from build123d import *

# Parameters (mm, degrees)
F0_W     = 10
F0_H     = 10
F0_W_2   = 8
F0_H_2   = 8
F1_DEPTH = 55
F2_R     = 1.5
F3_DEPTH = 25
F4_R     = 1.5
F5_DEPTH = 25


with BuildPart() as f1:
    # F0 (on Right) → F1 (new body)
    with BuildSketch(Plane.YZ):
        Rectangle(F0_W, F0_H)
        Rectangle(F0_W_2, F0_H_2, mode=Mode.SUBTRACT)
    extrude(amount=F1_DEPTH)

    # F2 (on face) → F3 (cut)
    with BuildSketch(Plane.XY.offset(5)):
        with Locations((5, 0)):
            Circle(F2_R)
        with Locations((50, 0)):
            Circle(F2_R)
    extrude(amount=-F3_DEPTH, mode=Mode.SUBTRACT)

    # F4 (on face) → F5 (cut)
    with BuildSketch(Plane.XZ.offset(5)):
        with Locations((15, 0)):
            Circle(F4_R)
        with Locations((40, 0)):
            Circle(F4_R)
    extrude(amount=-F5_DEPTH, mode=Mode.SUBTRACT)


solid = f1.part
Read the model definition and answer for the solid it produces. Units are mm, in the model's axes. A direction names the side the tool comes from. Give positions to 0.01 mm unless a question says otherwise; leave off trailing zeros. Write each loop counter-clockwise with the first axis right and the second up, starting at its lowest first coordinate (ties: lowest second). Pieces come first, ordered by that corner, then holes. Notation, with made-up numbers: (50.5, 55) - (91.5, 55) arc R15 cw to (91.5, 79) - close; hole circle Ø7 at (58.25, 57). An arc over 180 degrees is marked (long way). Use CSV: the item, a comma, the result in double quotes. Start each with the question number.
(1) Determine the mould class of faces 1 (the flat face through (27, -5, 0)), 2 (the cylindrical face through (13.5, 4.49, 0.07)), 3 (the flat face through (27, 0, 5)) for opening direction Z: +Z half, -Z half, draft (parallel to the pull), parting line (faces both ways), or undercut.
(2) Find section A-A (z = 0). Give the vertices of the cut face in (x, y).
(3) For faces 4 (the flat face through (27, 4, 0)), 5 (the flat face through (27, 0, -5)), determine the directions among +Z, -Z, +X, -X, +Y, -Y from which every point of the face is accessible in a straight line to the end or side of a thin tool.
(4) Find section B-B (x = 50). Give the vertices of the cut face in (y, z), plus the area to 3 significant figures.
(5) Given P1, Ø1.8, axis at x = 40, z = 0, coming from the -Y side, flat-ended and moving along its own axis, determine where the tip first touches the part or whether it passes through.
(6) Find section C-C (y = 0). Give the vertices of the cut face in (x, z).
(7) Find section D-D (z = -3). Give the vertices of the cut face in (x, y).
(8) Consider line 1 along Z through (x, y) = (34, 0); line 2 along X through (y, z) = (0.5, -4.25); line 3 along Z through (x, y) = (15, -4.5). Determine where each line is inside the solid, lowest interval first.
Findings below:
1,face 1,"draft"
1,face 2,"undercut"
1,face 3,"+Z half"
2,outline,"(0, -5) - (13.5, -5) - (13.5, -4) - (0, -4) - close; (0, 4) - (13.5, 4) - (13.5, 5) - (0, 5) - close; (16.5, -5) - (38.5, -5) - (38.5, -4) - (16.5, -4) - close; (16.5, 4) - (38.5, 4) - (38.5, 5) - (16.5, 5) - close; (41.5, -5) - (55, -5) - (55, -4) - (41.5, -4) - close; (41.5, 4) - (55, 4) - (55, 5) - (41.5, 5) - close"
3,face 4,"+X, -X"
3,face 5,"-Z, +X, -X, +Y, -Y"
4,outline,"(-5, -5) - (-1.5, -5) - (-1.5, -4) - (-4, -4) - (-4, 4) - (-1.5, 4) - (-1.5, 5) - (-5, 5) - close; (1.5, -5) - (5, -5) - (5, 5) - (1.5, 5) - (1.5, 4) - (4, 4) - (4, -4) - (1.5, -4) - close"
4,area,"30.0 mm2"
5,P1,"through"
6,outline,"(0, -5) - (3.5, -5) - (3.5, -4) - (0, -4) - close; (0, 4) - (3.5, 4) - (3.5, 5) - (0, 5) - close; (6.5, -5) - (48.5, -5) - (48.5, -4) - (6.5, -4) - close; (6.5, 4) - (48.5, 4) - (48.5, 5) - (6.5, 5) - close; (51.5, -5) - (55, -5) - (55, -4) - (51.5, -4) - close; (51.5, 4) - (55, 4) - (55, 5) - (51.5, 5) - close"
7,outline,"(0, -5) - (55, -5) - (55, -4) - (0, -4) - close; (0, 4) - (55, 4) - (55, 5) - (0, 5) - close"
8,line 1,"-5 to -4, 4 to 5"
8,line 2,"0 to 3.59, 6.41 to 48.59, 51.41 to 55"
8,line 3,"-5 to -1.5, 1.5 to 5"
